Source: CAD feature listing. Evaluate the final solid. Frame: model axes, mm. A direction names the side the tool comes from. Round coordinates to 2 decimals unless told otherwise and drop trailing zeros. Write each loop counter-clockwise with the first axis right and the second up, starting at its lowest first coordinate (ties: lowest second). Pieces come first, ordered by that corner, then holes. Notation, with made-up numbers: M -6,69.5 L 43,69.5 A14 ccw 43,86.5 Z; hole C 17.25,-17 d11. An arc over 180 degrees is marked long. Use a Markdown table: item, result.
```python
from build123d import *

# Parameters (mm, degrees)
EXTRUDE_1_DEPTH             = 25
EXTRUDE_2_DEPTH             = 12
EXTRUDE_3_DEPTH             = 3
SKETCH_4_W                  = 8
SKETCH_4_H                  = 3
CUT_EXTRUDE_1_DEPTH         = 41
SKETCH_5_W                  = 4.1
SKETCH_5_H                  = 39
SKETCH_6_W                  = 4.1
SKETCH_6_H                  = 39
SKETCH_7_W                  = 4.1
SKETCH_7_H                  = 39
SKETCH_8_W                  = 4.1
SKETCH_8_H                  = 39
SKETCH_9_W                  = 4.1
SKETCH_9_H                  = 39
SKETCH_10_W                 = 4.1
SKETCH_10_H                 = 39
HOLE_WIZARD_8_2_8_2_1_D     = 8.2
HOLE_WIZARD_8_2_8_2_1_DEPTH = 39
HOLE_WIZARD_8_2_8_2_2_D     = 8.2
HOLE_WIZARD_8_2_8_2_2_DEPTH = 14
HOLE_WIZARD_8_2_8_2_3_D     = 8.2
HOLE_WIZARD_8_2_8_2_3_DEPTH = 40
HOLE_WIZARD_4_5_4_5_1_D     = 4.5
HOLE_WIZARD_4_5_4_5_1_DEPTH = 40
HOLE_WIZARD_11_0_11_1_D     = 11
HOLE_WIZARD_11_0_11_1_DEPTH = 40
HOLE_WIZARD_10_0_10_1_D     = 10
HOLE_WIZARD_10_0_10_1_DEPTH = 40
HOLE_WIZARD_3_6_3_6_1_D     = 3.6
HOLE_WIZARD_3_6_3_6_1_DEPTH = 40
FILLET_1_R                  = 1
FILLET_2_R                  = 2
FILLET_3_R                  = 3


with BuildPart() as part:
    # 草图1 → 凸台-拉伸1 (new body)
    with BuildSketch(Plane.XY.offset(40)):
        with BuildLine():
            Line((-30.8, 160), (-30.8, 165))
            Line((-30.8, 165), (-42.426406871, 165))
            ThreePointArc((-42.426406871, 165), (-43.14973204, 162.7710855), (-43.756046661, 160.507539227))
            ThreePointArc((-43.756046661, 160.507539227), (-43.432520931, 159.373616076), (-42.294710456, 159.064039051))
            ThreePointArc((-42.294710456, 159.064039051), (-30.65, 150), (-42.294710456, 140.935960949))
            ThreePointArc((-42.294710456, 140.935960949), (-43.432520931, 140.626383924), (-43.756046661, 139.492460773))
            ThreePointArc((-43.756046661, 139.492460773), (-42.797543233, 136.094235253), (-41.575561951, 132.781618878))
            ThreePointArc((-41.575561951, 132.781618878), (-40.647320832, 132.054419431), (-39.544848012, 132.472754574))
            ThreePointArc((-39.544848012, 132.472754574), (-24.796370878, 131.984382017), (-28.889431051, 117.806831314))
            ThreePointArc((-28.889431051, 117.806831314), (-29.627974251, 116.887590023), (-29.22320876, 115.78006327))
            ThreePointArc((-29.22320876, 115.78006327), (-26.450336353, 113.594235253), (-23.514625677, 111.632534886))
            ThreePointArc((-23.514625677, 111.632534886), (-22.336225726, 111.589824616), (-21.690197707, 112.57628212))
            ThreePointArc((-21.690197707, 112.57628212), (-9.471370878, 120.850117776), (-4.449370899, 106.974397911))
            ThreePointArc((-4.449370899, 106.974397911), (-4.506548426, 105.796611284), (-3.528098373, 105.138518506))
            ThreePointArc((-3.528098373, 105.138518506), (0, 105), (3.528098373, 105.138518506))
            ThreePointArc((3.528098373, 105.138518506), (4.506548426, 105.796611284), (4.449370899, 106.974397911))
            ThreePointArc((4.449370899, 106.974397911), (9.471370878, 120.850117776), (21.690197707, 112.57628212))
            ThreePointArc((21.690197707, 112.57628212), (22.336225726, 111.589824616), (23.514625677, 111.632534886))
            ThreePointArc((23.514625677, 111.632534886), (26.450336353, 113.594235253), (29.22320876, 115.78006327))
            ThreePointArc((29.22320876, 115.78006327), (29.627974251, 116.887590023), (28.889431051, 117.806831314))
            ThreePointArc((28.889431051, 117.806831314), (24.796370878, 131.984382017), (39.544848012, 132.472754574))
            ThreePointArc((39.544848012, 132.472754574), (40.647320832, 132.054419431), (41.575561951, 132.781618878))
            ThreePointArc((41.575561951, 132.781618878), (42.797543233, 136.094235253), (43.756046661, 139.492460773))
            ThreePointArc((43.756046661, 139.492460773), (43.432520931, 140.626383924), (42.294710456, 140.935960949))
            ThreePointArc((42.294710456, 140.935960949), (30.65, 150), (42.294710456, 159.064039051))
            ThreePointArc((42.294710456, 159.064039051), (43.432520931, 159.373616076), (43.756046661, 160.507539227))
            ThreePointArc((43.756046661, 160.507539227), (43.14973204, 162.7710855), (42.426406871, 165))
            Line((42.426406871, 165), (30.8, 165))
            Line((30.8, 165), (30.8, 160))
            ThreePointArc((30.8, 160), (30.438925132, 157.230732571), (29.379844057, 154.646634192))
            ThreePointArc((29.379844057, 154.646634192), (28.022973878, 151.464418622), (27.431201542, 148.055988174))
            ThreePointArc((27.431201542, 148.055988174), (0, 122.5), (-27.431201542, 148.055988174))
            ThreePointArc((-27.431201542, 148.055988174), (-28.022973878, 151.464418622), (-29.379844057, 154.646634192))
            ThreePointArc((-29.379844057, 154.646634192), (-30.438925132, 157.230732571), (-30.8, 160))
        make_face()
    extrude(amount=-EXTRUDE_1_DEPTH)

    # 草图2 → 凸台-拉伸2 (add)
    with BuildSketch(Plane(origin=(0, 0, 15), x_dir=(-1, 0, 0), z_dir=(0, 0, -1))):
        with BuildLine():
            Line((-42.426406871, 165), (-30.8, 165))
            Line((-30.8, 165), (-30.8, 160))
            ThreePointArc((-30.8, 160), (-26.024303752, 151.036308556), (-15.920784389, 150))
            Line((-15.920784389, 150), (-11.5, 150))
            ThreePointArc((-11.5, 150), (0, 138.5), (11.5, 150))
            Line((11.5, 150), (15.920784389, 150))
            ThreePointArc((15.920784389, 150), (26.024303752, 151.036308556), (30.8, 160))
            Line((30.8, 160), (30.8, 165))
            Line((30.8, 165), (42.426406871, 165))
            ThreePointArc((42.426406871, 165), (43.14973204, 162.7710855), (43.756046661, 160.507539227))
            ThreePointArc((43.756046661, 160.507539227), (43.432520931, 159.373616076), (42.294710456, 159.064039051))
            ThreePointArc((42.294710456, 159.064039051), (30.65, 150), (42.294710456, 140.935960949))
            ThreePointArc((42.294710456, 140.935960949), (43.432520931, 140.626383924), (43.756046661, 139.492460773))
            ThreePointArc((43.756046661, 139.492460773), (42.797543233, 136.094235253), (41.575561951, 132.781618878))
            ThreePointArc((41.575561951, 132.781618878), (40.647320832, 132.054419431), (39.544848012, 132.472754574))
            ThreePointArc((39.544848012, 132.472754574), (24.796370878, 131.984382017), (28.889431051, 117.806831314))
            ThreePointArc((28.889431051, 117.806831314), (29.627974251, 116.887590023), (29.22320876, 115.78006327))
            ThreePointArc((29.22320876, 115.78006327), (26.450336353, 113.594235253), (23.514625677, 111.632534886))
            ThreePointArc((23.514625677, 111.632534886), (22.336225726, 111.589824616), (21.690197707, 112.57628212))
            ThreePointArc((21.690197707, 112.57628212), (9.471370878, 120.850117776), (4.449370899, 106.974397911))
            ThreePointArc((4.449370899, 106.974397911), (4.506548426, 105.796611284), (3.528098373, 105.138518506))
            ThreePointArc((3.528098373, 105.138518506), (0, 105), (-3.528098373, 105.138518506))
            ThreePointArc((-3.528098373, 105.138518506), (-4.506548426, 105.796611284), (-4.449370899, 106.974397911))
            ThreePointArc((-4.449370899, 106.974397911), (-9.471370878, 120.850117776), (-21.690197707, 112.57628212))
            ThreePointArc((-21.690197707, 112.57628212), (-22.336225726, 111.589824616), (-23.514625677, 111.632534886))
            ThreePointArc((-23.514625677, 111.632534886), (-26.450336353, 113.594235253), (-29.22320876, 115.78006327))
            ThreePointArc((-29.22320876, 115.78006327), (-29.627974251, 116.887590023), (-28.889431051, 117.806831314))
            ThreePointArc((-28.889431051, 117.806831314), (-24.796370878, 131.984382017), (-39.544848012, 132.472754574))
            ThreePointArc((-39.544848012, 132.472754574), (-40.647320832, 132.054419431), (-41.575561951, 132.781618878))
            ThreePointArc((-41.575561951, 132.781618878), (-42.797543233, 136.094235253), (-43.756046661, 139.492460773))
            ThreePointArc((-43.756046661, 139.492460773), (-43.432520931, 140.626383924), (-42.294710456, 140.935960949))
            ThreePointArc((-42.294710456, 140.935960949), (-30.65, 150), (-42.294710456, 159.064039051))
            ThreePointArc((-42.294710456, 159.064039051), (-43.432520931, 159.373616076), (-43.756046661, 160.507539227))
            ThreePointArc((-43.756046661, 160.507539227), (-43.14973204, 162.7710855), (-42.426406871, 165))
        make_face()
    extrude(amount=EXTRUDE_2_DEPTH)

    # 草图3 → 凸台-拉伸3 (add)
    with BuildSketch(Plane.XY.offset(3)):
        with BuildLine():
            Line((44.366203353, 170.8), (-44.366203353, 170.8))
            ThreePointArc((-44.366203353, 170.8), (0, 101), (44.366203353, 170.8))
        make_face()
    extrude(amount=-EXTRUDE_3_DEPTH)

    # 草图4 → 切除-拉伸1 (cut, through all)
    with BuildSketch(Plane(origin=(0, 0, 0), x_dir=(-1, 0, 0), z_dir=(0, 0, -1))):
        with Locations((0, 166.5)):
            Rectangle(SKETCH_4_W, SKETCH_4_H)
    extrude(amount=-CUT_EXTRUDE_1_DEPTH, mode=Mode.SUBTRACT)

    # 草图5 → 切除-旋转1 (revolve, cut)
    with BuildSketch(Plane(origin=(0, 144.5, 0), x_dir=(1, 0, 0), z_dir=(0, 1, 0))):
        with Locations((28.05, -20.5)):
            Rectangle(SKETCH_5_W, SKETCH_5_H)
    revolve(axis=Axis((26, 144.5, 1), (0, 0, 1)), mode=Mode.SUBTRACT)

    # 草图6 → 切除-旋转2 (revolve, cut)
    with BuildSketch(Plane(origin=(0, 136, 0), x_dir=(1, 0, 0), z_dir=(0, 1, 0))):
        with Locations((22.05, -20.5)):
            Rectangle(SKETCH_6_W, SKETCH_6_H)
    revolve(axis=Axis((20, 136, 1), (0, 0, 1)), mode=Mode.SUBTRACT)

    # 草图7 → 切除-旋转3 (revolve, cut)
    with BuildSketch(Plane(origin=(0, 127, 0), x_dir=(1, 0, 0), z_dir=(0, 1, 0))):
        with Locations((8.55, -20.5)):
            Rectangle(SKETCH_7_W, SKETCH_7_H)
    revolve(axis=Axis((6.5, 127, 1), (0, 0, 1)), mode=Mode.SUBTRACT)

    # 草图8 → 切除-旋转4 (revolve, cut)
    with BuildSketch(Plane(origin=(0, 127, 0), x_dir=(1, 0, 0), z_dir=(0, 1, 0))):
        with Locations((-4.45, -20.5)):
            Rectangle(SKETCH_8_W, SKETCH_8_H)
    revolve(axis=Axis((-6.5, 127, 1), (0, 0, 1)), mode=Mode.SUBTRACT)

    # 草图9 → 切除-旋转5 (revolve, cut)
    with BuildSketch(Plane(origin=(0, 136, 0), x_dir=(1, 0, 0), z_dir=(0, 1, 0))):
        with Locations((-17.95, -20.5)):
            Rectangle(SKETCH_9_W, SKETCH_9_H)
    revolve(axis=Axis((-20, 136, 1), (0, 0, 1)), mode=Mode.SUBTRACT)

    # 草图10 → 切除-旋转6 (revolve, cut)
    with BuildSketch(Plane(origin=(0, 144.5, 0), x_dir=(1, 0, 0), z_dir=(0, 1, 0))):
        with Locations((-23.95, -20.5)):
            Rectangle(SKETCH_10_W, SKETCH_10_H)
    revolve(axis=Axis((-26, 144.5, 1), (0, 0, 1)), mode=Mode.SUBTRACT)

    # Ø8.2 (8.2) 直径孔1
    with Locations(Plane.XY.offset(40)):
        with Locations((-16.5, 127), (16.5, 127)):
            Hole(HOLE_WIZARD_8_2_8_2_1_D / 2, depth=HOLE_WIZARD_8_2_8_2_1_DEPTH)

    # Ø8.2 (8.2) 直径孔2
    with Locations(Plane.XY.offset(15)):
        with Locations((0, 134), (10, 136), (16, 144.5), (-10, 136), (-16, 144.5)):
            Hole(HOLE_WIZARD_8_2_8_2_2_D / 2, depth=HOLE_WIZARD_8_2_8_2_2_DEPTH)

    # Ø8.2 (8.2) 直径孔3
    with Locations(Plane(origin=(0, 0, 0), x_dir=(-1, 0, 0), z_dir=(0, 0, -1))):
        with Locations((0, 120)):
            Hole(HOLE_WIZARD_8_2_8_2_3_D / 2, depth=HOLE_WIZARD_8_2_8_2_3_DEPTH)

    # Ø4.5 (4.5) 直径孔1
    with Locations(Plane(origin=(0, 0, 0), x_dir=(-1, 0, 0), z_dir=(0, 0, -1))):
        with Locations((-40, 150), (-32.360679775, 126.488589908), (-12.360679775, 111.957739348), (12.360679775, 111.957739348), (32.360679775, 126.488589908), (40, 150)):
            Hole(HOLE_WIZARD_4_5_4_5_1_D / 2, depth=HOLE_WIZARD_4_5_4_5_1_DEPTH)

    # Ø11.0 (11) 直径孔1
    with Locations(Plane(origin=(0, 0, 0), x_dir=(-1, 0, 0), z_dir=(0, 0, -1))):
        with Locations((0, 150)):
            Hole(HOLE_WIZARD_11_0_11_1_D / 2, depth=HOLE_WIZARD_11_0_11_1_DEPTH)

    # Ø10.0 (10) 直径孔1
    with Locations(Plane(origin=(0, 0, 0), x_dir=(-1, 0, 0), z_dir=(0, 0, -1))):
        with Locations((20, 160), (-20, 160)):
            Hole(HOLE_WIZARD_10_0_10_1_D / 2, depth=HOLE_WIZARD_10_0_10_1_DEPTH)

    # Ø3.6 (3.6) 直径孔1
    with Locations(Plane(origin=(0, 0, 0), x_dir=(-1, 0, 0), z_dir=(0, 0, -1))):
        with Locations((5.656854249, 155.656854249), (-7, 166.5), (7, 166.5), (5.656854249, 144.343145751), (-5.656854249, 144.343145751), (-5.656854249, 155.656854249)):
            Hole(HOLE_WIZARD_3_6_3_6_1_D / 2, depth=HOLE_WIZARD_3_6_3_6_1_DEPTH)

    # 圆角1
    fillet_1_edges = [part.edges().sort_by_distance(p)[0] for p in [
        (3.106287817, 122.676, 27.5),
        (-3.106287817, 122.676, 27.5),
    ]]
    fillet(fillet_1_edges, radius=FILLET_1_R)

    # 圆角2
    fillet_2_edges = [part.edges().sort_by_distance(p)[0] for p in [
        (-11.5, 150, 9),
        (11.5, 150, 9),
        (44.366203353, 170.8, 1.5),
        (-44.366203353, 170.8, 1.5),
    ]]
    fillet(fillet_2_edges, radius=FILLET_2_R)

    # 圆角3
    fillet_3_edges = [part.edges().sort_by_distance(p)[0] for p in [
        (30.8, 165, 21.5),
        (42.426406871, 165, 21.5),
        (-42.426406871, 165, 21.5),
        (-30.8, 165, 21.5),
    ]]
    fillet(fillet_3_edges, radius=FILLET_3_R)


solid = part.part
```
Q1. Line query: L1, parallel to Y at x = 0, z = 1.25; L2, parallel to X at y = 112, z = 19; L3, parallel to Y at x = -40.5, z = 20.5. Output: solid intervals per line, ascending.
Results are:
| item | result |
|---|---|
| L1 | 101 to 115.9, 124.1 to 129.9, 138.1 to 144.5, 155.5 to 165, 168 to 170.8 |
| L2 | -24.1 to -21.88, -3.01 to 3.01, 21.88 to 24.1 |
| L3 | 132.04 to 140.66, 159.34 to 164.99 |
Q2. First-contact query: pin 1 Ø11 at (x, y) = (32.36, 126.49) entering from +Z; pin 2 Ø5 at (y, z) = (121, 7.5) entering from +X; pin 3 Ø2.5 at (x, y) = (-26.5, 143) entering from +Z. Flat tips, straight axial feed; report the tip coordinate or a pass-through.
Results are:
| item | result |
|---|---|
| pin 1 | z = 3 |
| pin 2 | x = 27.5 |
| pin 3 | z = 1 |
Q3. Section B-B on x = 36. Return loops of the section in (y, z).
Results are:
| item | result |
|---|---|
| outline | M 116.76,0 L 170.8,0 L 170.8,3 L 165,3 L 165,40 L 158.45,40 L 158.45,3 L 141.55,3 L 141.55,40 L 135.1,40 L 135.1,3 L 116.76,3 Z |
Q4. Section A-A on x = 0. Return loops of the section in (y, z).
Results are:
| item | result |
|---|---|
| outline | M 101,0 L 115.9,0 L 115.9,40 L 105,40 L 105,3 L 101,3 Z; M 124.1,0 L 144.5,0 L 144.5,3 L 138.5,3 L 138.5,15 L 138.1,15 L 138.1,1 L 129.9,1 L 129.9,15 L 124.1,15 Z; M 155.5,0 L 165,0 L 165,3 L 155.5,3 Z; M 168,0 L 170.8,0 L 170.8,3 L 168,3 Z |
Q5. Reachability of faces 4 (the cylindrical face through (29.63, 116.87, 21.76)), 5 (the cylindrical face through (0, 105, 22)), 6 (the flat face through (-26, 145, 1)), 7 (the flat face through (37, 165, 22)) from +Z, -Z, +X, -X, +Y, -Y: full face, straight path, thin tool, end or side. Return the list, or none.
Results are:
| item | result |
|---|---|
| face 4 | +Z, +X |
| face 5 | +Z, -Y |
| face 6 | +Z |
| face 7 | +Z, +X, -X, +Y |
Q6. Mould query, pull axis Y, two halves, no side actions, for faces 1 (the cylindrical face through (26.41, 113.565, 21.759)), 2 (the flat face through (16, 145, 1)), 3 (the cylindrical face through (28.077, 151.643, 27.675)). Classes: +Y half, -Y half, draft (parallel to the pull), parting line (faces both ways), or undercut.
Results are:
| item | result |
|---|---|
| face 1 | -Y half |
| face 2 | undercut |
| face 3 | +Y half |
